Verification items for the finished model (mm, model axes). A direction names the side the tool comes from. Coordinates: 2 decimals unless noted, no trailing zeros. Write each loop counter-clockwise with the first axis right and the second up, starting at its lowest first coordinate (ties: lowest second). Pieces come first, ordered by that corner, then holes. Notation, with made-up numbers: (53.25, 28) - (98.25, 28) arc R19 cw to (98.25, 52) - close; hole circle Ø4 at (60.5, -13.75). An arc over 180 degrees is marked (long way). Answer as CSV lines item,"result". Start each with the question number.
```python
from build123d import *

# Parameters (mm, degrees)
SKETCH1_W             = 120.8024
SKETCH1_H             = 166.5224
BOSS_EXTRUDE1_DEPTH   = 5.7912
SKETCH7_R             = 1.30175
CUT_EXTRUDE6_DEPTH    = 104.025581213
SKETCH9_W             = 5.7912
SKETCH9_H             = 27.9908
CUT_EXTRUDE7_DEPTH    = 104.025581213
SKETCH10_W            = 5.7912
SKETCH10_H            = 27.516666666
CUT_EXTRUDE8_DEPTH    = 104.025581213
SKETCH11_R            = 1.30175
CUT_EXTRUDE9_DEPTH    = 104.025581213
SKETCH12_R            = 1.30175
CUT_EXTRUDE10_DEPTH   = 104.025581213
CAVITY2_START         = -83.2612
CAVITY2_OUTLINE_W     = 40.267466667
CAVITY2_OUTLINE_H     = 5.7912
CAVITY2_DEPTH         = 5.7912
CAVITY2_START_2       = 77.47
CAVITY2_2_OUTLINE_W   = 40.267466667
CAVITY2_2_OUTLINE_H   = 5.7912
CAVITY2_2_OUTLINE_W_2 = 34.476266667
CAVITY2_2_DEPTH       = 5.7912
CAVITY2_START_3       = -27.2796
CAVITY2_3_OUTLINE_W   = 5.7912
CAVITY2_3_OUTLINE_H   = 5.7912
CAVITY2_3_DEPTH       = 55.507466667
CAVITY2_START_4       = -77.47
CAVITY2_4_OUTLINE_W   = 5.7912
CAVITY2_4_OUTLINE_H   = 5.7912
CAVITY2_4_DEPTH       = 22.1996
CAVITY2_START_5       = 55.744533333
CAVITY2_5_OUTLINE_W   = 5.7912
CAVITY2_5_OUTLINE_H   = 5.7912
CAVITY2_5_DEPTH       = 21.725466667


# Read off the part's stored shape, not the designer's step: Cavity2
with BuildPart() as part:
    # Sketch1 → Boss-Extrude1 (new body)
    with BuildSketch(Plane.XY):
        Rectangle(SKETCH1_W, SKETCH1_H)
    extrude(amount=BOSS_EXTRUDE1_DEPTH)

    # Sketch7 → Cut-Extrude6 (cut, through all)
    with BuildSketch(Plane.XY.offset(5.7912)):
        with Locations((-57.5056, -41.275)):
            Circle(SKETCH7_R)
        with Locations((-57.5056, 41.9862)):
            Circle(SKETCH7_R)
        with Locations(Location((58.473654732, -41.275, 0), (0, 0, 180))):
            Circle(SKETCH7_R)
        with Locations(Location((58.473654732, 41.9862, 0), (0, 0, 180))):
            Circle(SKETCH7_R)
    extrude(amount=-CUT_EXTRUDE6_DEPTH, mode=Mode.SUBTRACT)

    # Sketch9 → Cut-Extrude7 (cut, through all)
    with BuildSketch(Plane.XY.offset(5.7912)):
        with Locations((57.5056, -41.275)):
            Rectangle(SKETCH9_W, SKETCH9_H)
    extrude(amount=-CUT_EXTRUDE7_DEPTH, mode=Mode.SUBTRACT)

    # Sketch10 → Cut-Extrude8 (cut, through all)
    with BuildSketch(Plane.XY.offset(5.7912)):
        with Locations((57.5056, 41.9862)):
            Rectangle(SKETCH10_W, SKETCH10_H)
    extrude(amount=-CUT_EXTRUDE8_DEPTH, mode=Mode.SUBTRACT)

    # Sketch11 → Cut-Extrude9 (cut, through all)
    with BuildSketch(Plane.XY.offset(5.7912)):
        with Locations((57.5056, 0.474133333)):
            Circle(SKETCH11_R)
    extrude(amount=-CUT_EXTRUDE9_DEPTH, mode=Mode.SUBTRACT)

    # Sketch12 → Cut-Extrude10 (cut, through all)
    with BuildSketch(Plane.XY.offset(5.7912)):
        with Locations((0, 80.3656)):
            Circle(SKETCH12_R)
        with Locations((0, -80.3656)):
            Circle(SKETCH12_R)
    extrude(amount=-CUT_EXTRUDE10_DEPTH, mode=Mode.SUBTRACT)

    # Cavity2 outline → Cavity2 (cut)
    with BuildSketch(Plane(origin=(0, 0, 0), x_dir=(1, 0, 0), z_dir=(0, 1, 0)).offset(CAVITY2_START)):
        with Locations((-40.267466666, -2.8956)):
            Rectangle(CAVITY2_OUTLINE_W, CAVITY2_OUTLINE_H)
        with Locations((40.267466666, -2.8956)):
            Rectangle(CAVITY2_OUTLINE_W, CAVITY2_OUTLINE_H)
    extrude(amount=CAVITY2_DEPTH, mode=Mode.SUBTRACT)

    # Cavity2 2 outline → Cavity2 2 (cut)
    with BuildSketch(Plane(origin=(0, 0, 0), x_dir=(1, 0, 0), z_dir=(0, 1, 0)).offset(CAVITY2_START_2)):
        with Locations((-40.267466666, -2.8956)):
            Rectangle(CAVITY2_2_OUTLINE_W, CAVITY2_2_OUTLINE_H)
        with Locations((37.371866667, -2.8956)):
            Rectangle(CAVITY2_2_OUTLINE_W_2, CAVITY2_2_OUTLINE_H)
    extrude(amount=CAVITY2_2_DEPTH, mode=Mode.SUBTRACT)

    # Cavity2 3 outline → Cavity2 3 (cut)
    with BuildSketch(Plane(origin=(0, 0, 0), x_dir=(1, 0, 0), z_dir=(0, 1, 0)).offset(CAVITY2_START_3)):
        with Locations((-57.5056, -2.8956)):
            Rectangle(CAVITY2_3_OUTLINE_W, CAVITY2_3_OUTLINE_H)
    extrude(amount=CAVITY2_3_DEPTH, mode=Mode.SUBTRACT)

    # Cavity2 4 outline → Cavity2 4 (cut)
    with BuildSketch(Plane(origin=(0, 0, 0), x_dir=(1, 0, 0), z_dir=(0, 1, 0)).offset(CAVITY2_START_4)):
        with Locations((-57.5056, -2.8956)):
            Rectangle(CAVITY2_4_OUTLINE_W, CAVITY2_4_OUTLINE_H)
    extrude(amount=CAVITY2_4_DEPTH, mode=Mode.SUBTRACT)

    # Cavity2 5 outline → Cavity2 5 (cut)
    with BuildSketch(Plane(origin=(0, 0, 0), x_dir=(1, 0, 0), z_dir=(0, 1, 0)).offset(CAVITY2_START_5)):
        with Locations((-57.5056, -2.8956)):
            Rectangle(CAVITY2_5_OUTLINE_W, CAVITY2_5_OUTLINE_H)
    extrude(amount=CAVITY2_5_DEPTH, mode=Mode.SUBTRACT)


solid = part.part
```
1. Depth check by flat-ended pin: P1, Ø3, axis at y = 80, z = 2, coming from the -X side; P2, Ø1.5, axis at y = -34, z = 2, coming from the +X side; P3, Ø3, axis at x = 44.5, z = 4.5, coming from the -Y side. Enter the tip coordinate at first touch or a pass-through.
2. Access from +Z, -Z, +X, -X, +Y, -Y to the whole of each face (thin tool, end or side, straight path). Record for faces 1 (the face through (-58, -27.28, 3)), 2 (the face through (-54.61, -67, 3)), 3 (the face through (-20.134, 80, 3)), 4 (the face through (57, 55.745, 3)), 5 (the face through (20.134, 80, 3)).
3. Scan lines: line 1 along Y through (x, z) = (0, 3.25); line 2 along X through (y, z) = (-35, 4.4); line 3 along Y through (x, z) = (37, 0.4). Record each from-to range of solid material in increasing order. Write a range as from..to.
4. Cross-section at A-A (y = 37). Record the cut outline in (x, z).
5. Draft check along X on faces 6 (the face through (0, -83.261, 3)), 7 (the face through (-54.61, 0, 3)), 8 (the face through (54.61, 80, 3)). Enter one of: pulls with the +X half, pulls with the -X half, needs draft (parallel to the pull), parting line crosses it, or undercut.
6. Cross-section at C-C (z = 2.95). Count the separate pieces of the cut face and the enclosed holes in it, and give its area (3 significant figures).
7. Cross-section at B-B (x = 41.5). Record the cut outline in (y, z).
Completed:
1,P1,"stops at x = -20.13"
1,P2,"stops at x = 54.61"
1,P3,"stops at y = -77.47"
2,face 1,"+Z, -Z, -X"
2,face 2,"+Z, -Z, -X, -Y"
2,face 3,"+Z, -Z, -X, +Y"
2,face 4,"+Z, -Z, +X"
2,face 5,"+Z, -Z, +Y"
3,line 1,"y = -83.26..-81.67, -79.06..79.06, 81.67..83.26"
3,line 2,"x = -60.4..54.61"
3,line 3,"y = -77.47..77.47"
4,outline,"(-60.4, 0) - (54.61, 0) - (54.61, 5.79) - (-60.4, 5.79) - close"
5,face 6,"needs draft"
5,face 7,"pulls with the -X half"
5,face 8,"undercut"
6,separate pieces,"1"
6,enclosed holes,"5"
6,area,"18,300 mm2"
7,outline,"(-77.47, 0) - (77.47, 0) - (77.47, 5.79) - (-77.47, 5.79) - close"
